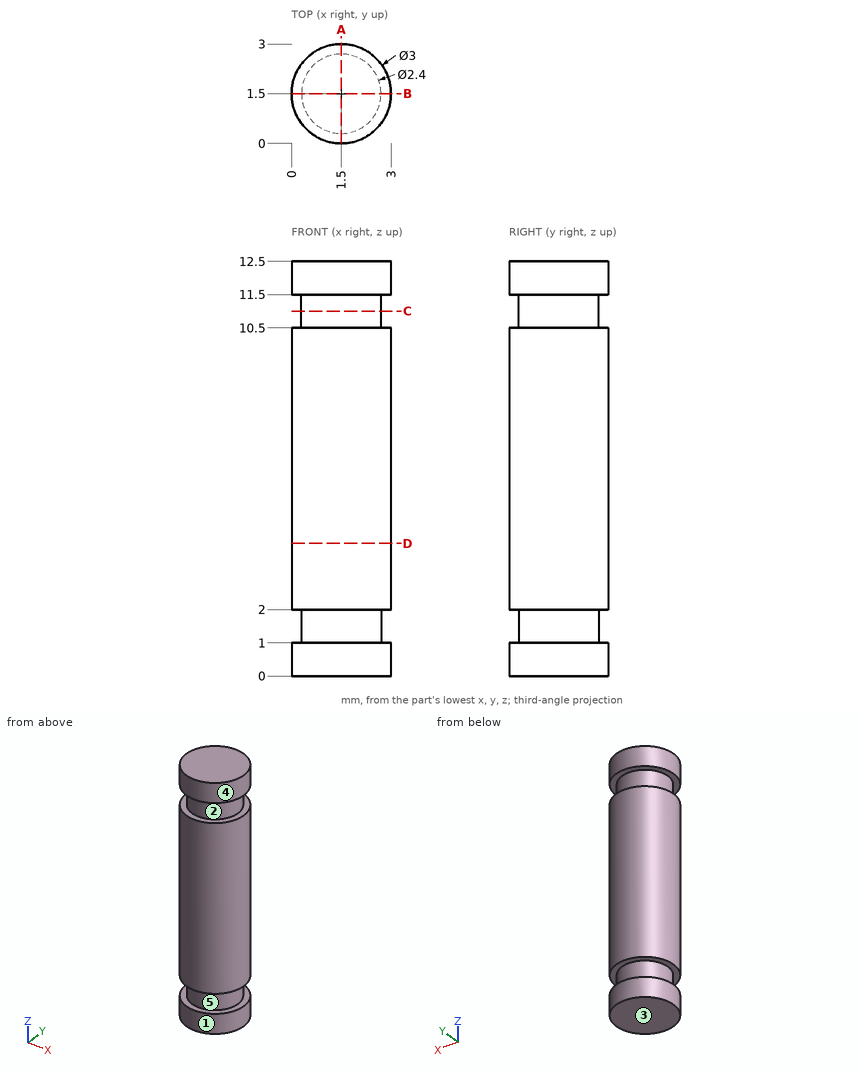
Print and shaded views of the part. All mm, measured from the part's lowest x, y and z. A direction names the side the tool comes from. Coordinates: 2 decimals unless noted, no trailing zeros. Write each loop counter-clockwise with the first axis right and the second up, starting at its lowest first coordinate (ties: lowest second). Pieces come first, ordered by that corner, then holes.
(1) Two-plate mould, pull along Z, no slides. Class the marked faces 1, 2 and 3: +Z half, -Z half, draft (parallel to the pull), parting line (faces both ways), or undercut.
(2) Cut at D-D, the plane z = 4. List the corners of the cut face in (x, y).
(3) Flat gauge pins, fed straight in: pin 1 (0.9 mm diameter, centred on x = 2, y = 1, fed in from -Z); pin 2 (1 mm diameter, centred on y = 2.5, z = 9, fed in from -X); pin 3 (1.5 mm diameter, centred on x = 0.5, z = 7.5, fed in from -Y). Where does each tip first touch, or does it go through?
(4) 3-axis set-ups, long thin cutter, end or side, ignore diameter. For the marked faces 4 and 5: which of +Z, -Z, +X, -X, +Y, -Y reach the whole face in a straight line?
(5) Drill centre lines: probe 1 along Z at (x, y) = (2.5, 0.65); probe 2 along X at (y, z) = (2.4, 0.5); probe 3 along X at (y, z) = (1.6, 4.25). Where is each one in solid material? Low to high.
(6) Cut at C-C, the plane z = 11. List the corners of the cut face in (x, y).
(7) Cut at A-A, the plane x = 1.5. List the corners of the cut face in (y, z), and give its area (3 significant figures).
Geometry says:
1. face 1: draft
1. face 2: undercut
1. face 3: -Z half
2. outline: circle Ø3 at (1.5, 1.5)
3. pin 1: stops at z = 0
3. pin 2: stops at x = 0.09
3. pin 3: stops at y = 0.02
4. face 4: +Z, -Z
4. face 5: none
5. probe 1: z = 0 to 1, 2 to 10.5, 11.5 to 12.5
5. probe 2: x = 0.3 to 2.7
5. probe 3: x = 0 to 3
6. outline: circle Ø2.4 at (1.5, 1.5)
7. outline: (0, 0) - (3, 0) - (3, 1) - (2.7, 1) - (2.7, 2) - (3, 2) - (3, 10.5) - (2.7, 10.5) - (2.7, 11.5) - (3, 11.5) - (3, 12.5) - (0, 12.5) - (0, 11.5) - (0.3, 11.5) - (0.3, 10.5) - (0, 10.5) - (0, 2) - (0.3, 2) - (0.3, 1) - (0, 1) - close
7. area: 36.3 mm2
